from build123d import *

# Parameters (mm, degrees)
SKETCH1_R           = 6.35
BOSS_EXTRUDE1_DEPTH = 28.575
SKETCH2_R           = 2.9464
CUT_EXTRUDE1_DEPTH  = 12.7
CUT_EXTRUDE2_START  = -5.08
SKETCH4_W           = 3.175
SKETCH4_H           = 3.175
CUT_EXTRUDE2_DEPTH  = 5.08


with BuildPart() as part:
    # Sketch1 → Boss-Extrude1 (new body)
    with BuildSketch(Plane.XY):
        Circle(SKETCH1_R)
    extrude(amount=BOSS_EXTRUDE1_DEPTH)

    # Sketch2 → Cut-Extrude1 (cut)
    with BuildSketch(Plane(origin=(0, 0, 0), x_dir=(-1, 0, 0), z_dir=(0, 0, -1))):
        Circle(SKETCH2_R)
    extrude(amount=-CUT_EXTRUDE1_DEPTH, mode=Mode.SUBTRACT)

    # Sketch4 → Cut-Extrude2 (cut)
    with BuildSketch(Plane.XY.offset(28.575).offset(CUT_EXTRUDE2_START)):
        with BuildLine():
            Line((-1.5875, 6.148361062), (-1.5875, 1.5875))
            Line((-1.5875, 1.5875), (1.5875, 1.5875))
            Line((1.5875, 1.5875), (1.5875, 6.148361062))
            ThreePointArc((1.5875, 6.148361062), (0, 6.35), (-1.5875, 6.148361062))
        make_face()
        Rectangle(SKETCH4_W, SKETCH4_H)
        with BuildLine():
            Line((-6.148361062, -1.5875), (-1.5875, -1.5875))
            Line((-1.5875, -1.5875), (-1.5875, 1.5875))
            Line((-1.5875, 1.5875), (-6.148361062, 1.5875))
            ThreePointArc((-6.148361062, 1.5875), (-6.35, 0), (-6.148361062, -1.5875))
        make_face()
        with BuildLine():
            Line((1.5875, 1.5875), (1.5875, -1.5875))
            Line((1.5875, -1.5875), (6.148361062, -1.5875))
            ThreePointArc((6.148361062, -1.5875), (6.299388571, -0.800127257), (6.35, 0))
            ThreePointArc((6.35, 0), (6.299388571, 0.800127257), (6.148361062, 1.5875))
            Line((6.148361062, 1.5875), (1.5875, 1.5875))
        make_face()
        with BuildLine():
            Line((-1.5875, -1.5875), (-1.5875, -6.148361062))
            ThreePointArc((-1.5875, -6.148361062), (0, -6.35), (1.5875, -6.148361062))
            Line((1.5875, -6.148361062), (1.5875, -1.5875))
            Line((1.5875, -1.5875), (-1.5875, -1.5875))
        make_face()
    extrude(amount=CUT_EXTRUDE2_DEPTH, mode=Mode.SUBTRACT)


solid = part.part
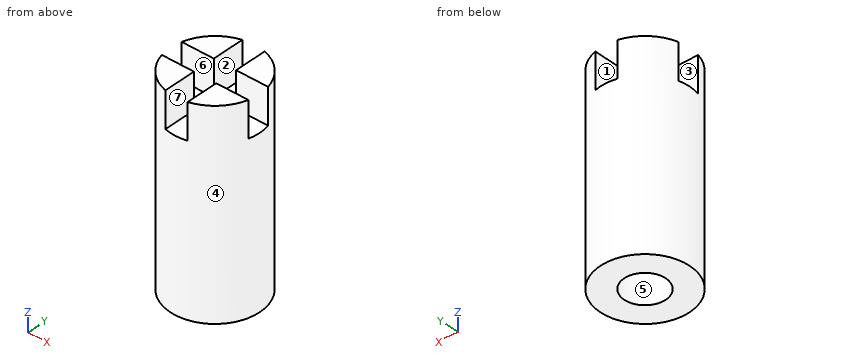
Read the model definition and answer for the solid it produces. Units are mm, in the model's axes. Face numbers are marked on the shaded views. A direction names the side the tool comes from. Coordinates: 2 decimals unless noted, no trailing zeros. Loops run counter-clockwise (first coordinate to the right, second up) from the corner with the lowest first, then second, coordinate; pieces in that order, holes last.
Q1. Which of the six approach directions +Z, -Z, +X, -X, +Y, -Y give full straight-line access (tool end or side, diameter ignored) to the marked faces 5, 6 and 7?
Q2. The part is cut by section A-A on y = 0. Write down the section's boundary in (x, z) (3 decimals).
Q3. The part is cut by section C-C on z = 9.75. Write down the section's boundary in (x, y).
Q4. The part is cut by section D-D on x = 2.5. Write down the section's boundary in (y, z) (1 decimal).
Q5. Consider probe 1 along Y at (x, z) = (0, 8.75); probe 2 along Z at (x, y) = (-2.5, 0.5) (3 decimals); probe 3 along Z at (x, y) = (-3, 1) (3 decimals). Determine where each line is inside the solid, lowest interval first.
Q6. Each of these flat-tipped pins is pushed along its axis until it touches: pin 1 Ø2.5 at (y, z) = (3, 25.5) entering from -X; pin 2 Ø3.5 at (x, z) = (-5, 27) entering from -Y; pin 3 Ø2.5 at (x, z) = (-5, 26) entering from +Y. Where does it stop, or does it pass through?
Q7. The mould has two halves that part along X. Classify the marked faces 1, 2, 3 and 4: +X half, -X half, draft (parallel to the pull), parting line (faces both ways), or undercut.
Results below:
1. face 5: -Z
1. face 6: +Z, +X, -X
1. face 7: +Z, +Y, -Y
2. outline: (-6.35, 0) - (-2.946, 0) - (-2.946, 12.7) - (2.946, 12.7) - (2.946, 0) - (6.35, 0) - (6.35, 23.495) - (-6.35, 23.495) - close
3. outline: circle Ø12.7 at (0, 0); hole circle Ø5.89 at (0, 0)
4. outline: (-5.8, 0) - (-1.6, 0) - (-1.6, 12.7) - (1.6, 12.7) - (1.6, 0) - (5.8, 0) - (5.8, 28.6) - (1.6, 28.6) - (1.6, 23.5) - (-1.6, 23.5) - (-1.6, 28.6) - (-5.8, 28.6) - close
5. probe 1: y = -6.35 to -2.95, 2.95 to 6.35
5. probe 2: z = 12.7 to 23.495
5. probe 3: z = 0 to 23.495
6. pin 1: stops at x = -6.1
6. pin 2: stops at y = -5.46
6. pin 3: stops at y = 5.12
7. face 1: undercut
7. face 2: undercut
7. face 3: draft
7. face 4: parting line
